The drawing under review shows one solid part. Ordinate dimensions are in mm from its lowest x, y, z. A direction names the side the tool comes from. Coordinates: 2 decimals unless noted, no trailing zeros. Write each loop counter-clockwise with the first axis right and the second up, starting at its lowest first coordinate (ties: lowest second). Pieces come first, ordered by that corner, then holes.
1) Add section C-C, the plane z = 3.3. State the section outline as (x, y) points, then the cut area to 3 significant figures.
2) For P1, Ø2, axis at x = 4, z = 2, coming from the +Y side; P2, Ø3, axis at y = 5.5, z = 2, coming from the +X side; P3, Ø1, axis at x = 2.5, z = 1, coming from the +Y side, all flat-tipped, find the tip position at first contact; note any pin that passes through.
3) For line 1 (X direction, y = 11.75, z = 0.45); line 2 (Y direction, x = 8.5, z = 5.8); line 3 (Y direction, x = 5.75, z = 0.4), list the stretches that pass through material, from the lowest coordinate up.
4) Mouldability with a two-part tool opening along X and no side actions: class the marked faces 1, 2 and 3 as released by +X, released by -X, zero draft, split by the parting line, or undercut.
5) Machinability: for the marked faces 4, 5 and 6, which of the approach directions +Z, -Z, +X, -X, +Y, -Y give a long, thin tool a straight path to every point of the face, cutting with its end or side? Answer none if there is none.
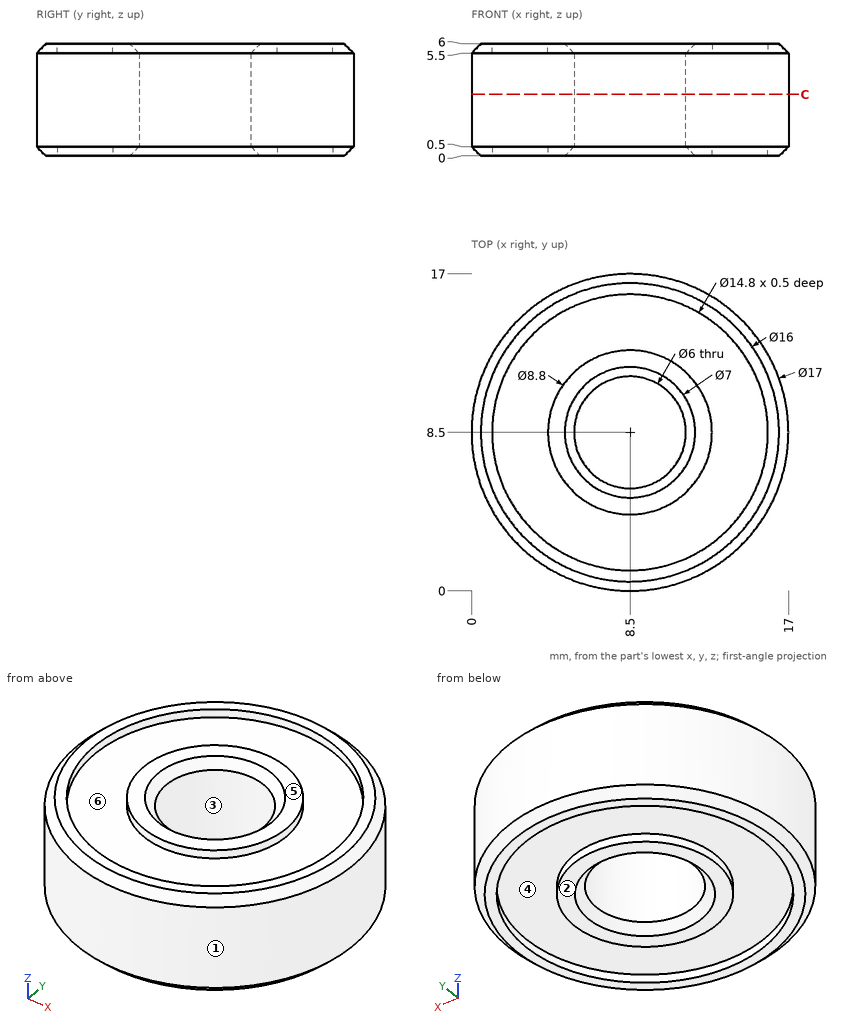
Geometry results:
1. outline: circle Ø17 at (8.5, 8.5); hole circle Ø6 at (8.5, 8.5)
1. area: 199 mm2
2. P1: stops at y = 16.25
2. P2: stops at x = 16.87
2. P3: stops at y = 14.98
3. line 1: x = 0.7 to 1.85, 5.53 to 11.47, 15.15 to 16.3
3. line 2: y = 0.3 to 1.1, 4.1 to 5.2, 11.8 to 12.9, 15.9 to 16.7
3. line 3: y = 0.56 to 1.63, 5.07 to 7.07, 9.93 to 11.93, 15.37 to 16.44
4. face 1: split by the parting line
4. face 2: zero draft
4. face 3: undercut
5. face 4: -Z
5. face 5: +Z, +X, -X, +Y, -Y
5. face 6: +Z
